Verification items for the finished model (mm, model axes). A direction names the side the tool comes from. Give positions to 0.01 mm unless a question says otherwise; leave off trailing zeros. Order: outer loops, then holes, each group sorted by start corner. A loop starts at its lowest first (then second) coordinate and runs counter-clockwise, first axis right, second up. Notation, with made-up numbers: (7, -2) - (51, -2) arc R32 cw to (51, 26) - close; hole circle Ø8 at (64.5, -3). An arc over 180 degrees is marked (long way). Answer as a JSON object with one key per item and string values. Group by question number.
(1) Thickness scan on line 1 (Z direction, x = 5.5, y = 39.3); line 2 (Z direction, x = 39, y = 3); line 3 (Y direction, x = 11, z = -11). Record the ranges inside material, lowest first.
(2) Access from +Z, -Z, +X, -X, +Y, -Y to the whole of each face (thin tool, end or side, straight path). Record for faces 1 (the face through (1.9, 36, 2)), 2 (the face through (21, 15, 2.4)), 3 (the face through (21, -2.4, -7)), 4 (the face through (21, 20, 0)), 5 (the face through (38.95, 40.28, 2.55)).
(3) Mould release check, pull along X, two halves, no side actions. Record for faces 6 (the face through (3.45, 40.28, 2.48)), 7 (the face through (40.5, 36, 2)), 8 (the face through (20.9, -1.8, 1.83)), 9 (the face through (10, 39, 2)): +X half, -X half, draft (parallel to the pull), parting line (faces both ways), or undercut.
(4) Section check B-B (x = 6). Record the boundary of the cut face in (y, z).
(5) Depth check by flat-ended pin: pin 1 Ø2 at (x, z) = (20, 2.5) entering from -Y; pin 2 Ø3.5 at (y, z) = (39, 3.5) entering from -X; pin 3 Ø10 at (x, z) = (23.5, -3.5) entering from +Y. Enter the tip coordinate at first touch or a pass-through.
(6) Section check A-A (z = 3.73). Record the boundary of the cut face in (x, y), then the cut area to 3 significant figures.
(7) Section check D-D (y = 5). Record the boundary of the cut face in (x, z), then the cut area to 3 significant figures.
(8) Section check C-C (x = 11). Record the boundary of the cut face in (y, z).
```python
from build123d import *

# Parameters (mm, degrees)
SKETCH1_W           = 42.4
SKETCH1_H           = 40.6
BOSS_EXTRUDE1_DEPTH = 2.4
SKETCH2_W           = 40
SKETCH2_H           = 2.4
BOSS_EXTRUDE2_DEPTH = 17.35
SKETCH3_W           = 22.4
SKETCH3_H           = 2.6
CUT_EXTRUDE1_DEPTH  = 2.4
BOSS_EXTRUDE3_DEPTH = 2.53
FILLET1_R           = 5.25
FILLET2_R           = 5.25
CUT_EXTRUDE2_DEPTH  = 16.4
FILLET3_R           = 2
CHAMFER1_SIZE       = 2
SKETCH9_W           = 1.9
SKETCH9_H           = 10
CUT_EXTRUDE4_DEPTH  = 61.577409156
FILLET5_R           = 2
BOSS_EXTRUDE4_DEPTH = 2.4
CUT_EXTRUDE5_START  = -8.1
SKETCH4_R           = 0.8255
CUT_EXTRUDE5_DEPTH  = 38.6


with BuildPart() as part:
    # Sketch1 → Boss-Extrude1 (new body)
    with BuildSketch(Plane.XY):
        with Locations((21.2, 20.3)):
            Rectangle(SKETCH1_W, SKETCH1_H)
    extrude(amount=BOSS_EXTRUDE1_DEPTH)

    # Sketch2 → Boss-Extrude2 (add)
    with BuildSketch(Plane.XY.offset(2.4)):
        with Locations((20, -1.2)):
            Rectangle(SKETCH2_W, SKETCH2_H)
    extrude(amount=-BOSS_EXTRUDE2_DEPTH)

    # Sketch3 → Cut-Extrude1 (cut)
    with BuildSketch(Plane.XY.offset(2.4)):
        with Locations((21.2, 39.3)):
            Rectangle(SKETCH3_W, SKETCH3_H)
    extrude(amount=-CUT_EXTRUDE1_DEPTH, mode=Mode.SUBTRACT)

    # Sketch5 → Boss-Extrude3 (add)
    with BuildSketch(Plane.XY.offset(2.4)):
        Polygon((0, 40.6), (0, 34.6), (42.4, 34.6), (42.4, 40.6), (32.4, 40.6), (32.4, 38), (10, 38), (10, 40.6), align=None)
    extrude(amount=BOSS_EXTRUDE3_DEPTH)

    # Fillet1
    fillet1_edges = [part.edges().sort_by_distance(p)[0] for p in [
        (0, 40.6, 2.465),
        (42.4, 40.6, 2.465),
    ]]
    fillet(fillet1_edges, radius=FILLET1_R)

    # Fillet2
    # the kernel refuses this fillet: 5.25 mm, written as the material it adds along each edge
    with BuildSketch(Plane(origin=(0, 34.6, 2.4), x_dir=(0, 0, 1), z_dir=(1, 0, 0))) as fillet2_piece_1:
        with BuildLine():
            CenterArc((5.25, 4.490445412), FILLET2_R, 180, 58.795429652)
            Line((0, 4.490445412), (-0.105, 4.490445412))
            Line((-0.105, 4.490445412), (-0.105, 0))
            Line((-0.105, 0), (0, -0.105))
            ThreePointArc((0, -0.105), (1.265, -0.105), (2.4756, -0.089808908))
            Line((2.4756, -0.089808908), (2.53, 0))
        make_face()
    extrude(amount=42.4)

    # Sketch6 → Cut-Extrude2 (cut)
    with BuildSketch(Plane.ZY.offset(-32.4)):
        Polygon((0, 40.6), (0, 38.6), (0.25, 40.6), align=None)
    cut_extrude2 = extrude(amount=-CUT_EXTRUDE2_DEPTH, mode=Mode.SUBTRACT)

    # Fillet3
    fillet3_edges = [part.edges().sort_by_distance(p)[0] for p in [
        (20, -2.4, 2.4),
    ]]
    fillet(fillet3_edges, radius=FILLET3_R)

    # Chamfer1
    chamfer1_edges = [part.edges().sort_by_distance(p)[0] for p in [
        (21.2, 38, 4.93),
    ]]
    chamfer(chamfer1_edges, length=CHAMFER1_SIZE)

    # Sketch9 → Cut-Extrude4 (cut, through all)
    with BuildSketch(Plane(origin=(0, 0, 0), x_dir=(-1, 0, 0), z_dir=(0, 0, -1))):
        with Locations((-41.45, 35.6)):
            Rectangle(SKETCH9_W, SKETCH9_H)
        with Locations((-0.95, 35.6)):
            Rectangle(SKETCH9_W, SKETCH9_H)
    extrude(amount=-CUT_EXTRUDE4_DEPTH, mode=Mode.SUBTRACT)

    # Fillet5
    # the kernel refuses this fillet: 2 mm, written as the material it adds along each edge
    with BuildSketch(Plane(origin=(1.9, 30.6, 0), x_dir=(0, 1, 0), z_dir=(0, 0, 1))) as fillet5_piece_1_section:
        with BuildLine():
            CenterArc((1.997498436, 2), FILLET5_R, 182.865983983, 87.134016017)
            Line((0, 1.9), (-0.039949969, 1.898))
            ThreePointArc((-0.039949969, 1.898), (-0.04, 0.95), (-0.04, 0))
            Line((-0.04, 0), (0, -0.04))
            Line((0, -0.04), (1.997498436, -0.04))
            Line((1.997498436, -0.04), (1.997498436, 0))
        make_face()
    fillet5_piece_1 = extrude(amount=7.416704545, mode=Mode.PRIVATE)
    fillet5_piece_1 = fillet5_piece_1 - Plane(origin=(1.464355644, 30.109554588, 7.65), x_dir=(0, 0, 1), z_dir=(-1, 0, 0)) * Cylinder(5.25, 23, mode=Mode.PRIVATE)
    add(fillet5_piece_1)
    with BuildSketch(Plane(origin=(40.5, 30.6, 0), x_dir=(0, 1, 0), z_dir=(0, 0, 1))) as fillet5_piece_2_section:
        with BuildLine():
            CenterArc((1.997498436, -2), FILLET5_R, 90, 87.134016017)
            Line((0, -1.9), (-0.039949969, -1.898))
            ThreePointArc((-0.039949969, -1.898), (-0.04, -0.95), (-0.04, 0))
            Line((-0.04, 0), (0, 0.04))
            Line((0, 0.04), (1.997498436, 0.04))
            Line((1.997498436, 0.04), (1.997498436, 0))
        make_face()
    fillet5_piece_2 = extrude(amount=7.416704545, mode=Mode.PRIVATE)
    fillet5_piece_2 = fillet5_piece_2 - Plane(origin=(40.935644356, 30.109554588, 7.65), x_dir=(0, 0, 1), z_dir=(-1, 0, 0)) * Cylinder(5.25, 23, mode=Mode.PRIVATE)
    add(fillet5_piece_2)

    # Sketch10 → Boss-Extrude4 (add)
    with BuildSketch(Plane(origin=(40, 0, 0), x_dir=(0, 0, -1), z_dir=(1, 0, 0))):
        with BuildLine():
            Line((-2.4, 0), (-2.4, -0.4))
            ThreePointArc((-2.4, -0.4), (-1.814213562, -1.814213562), (-0.4, -2.4))
            Line((-0.4, -2.4), (14.95, -2.4))
            Line((14.95, -2.4), (14.95, 0))
            Line((14.95, 0), (0, 0))
            Line((0, 0), (-2.4, 0))
        make_face()
    extrude(amount=BOSS_EXTRUDE4_DEPTH)

    # Mirror1: Cut-Extrude2 across plane
    add(cut_extrude2.mirror(Plane(origin=(21.2, 0, 0), x_dir=(0, 0, 1), z_dir=(1, 0, 0))), mode=Mode.SUBTRACT)

    # Sketch4 → Cut-Extrude5 (cut)
    with BuildSketch(Plane(origin=(10, 0, 0), x_dir=(0, 0, -1), z_dir=(1, 0, 0)).offset(CUT_EXTRUDE5_START)):
        with Locations(Location((-3.73, 39.3, 0), (0, 0, 173.581911643))):
            Circle(SKETCH4_R)
    extrude(amount=CUT_EXTRUDE5_DEPTH, mode=Mode.SUBTRACT)


solid = part.part
```
Solutions:
{
 "1": {"line 1": "z = 0.09 to 2.9, 4.56 to 4.93", "line 2": "z = 0 to 2.4", "line 3": "y = -2.4 to 0"},
 "2": {"face 1": "+Z, -Z, -X, +Y", "face 2": "+Z, +X, -X, -Y", "face 3": "+Z, -Z, +X, -X, -Y", "face 4": "-Z, +X, -X, +Y", "face 5": "+Z, -Z, +X, +Y"},
 "3": {"face 6": "-X half", "face 7": "+X half", "face 8": "draft", "face 9": "undercut"},
 "4": {"outline": "(-2.4, -14.95) - (0, -14.95) - (0, 0) - (38.6, 0) - (40.6, 0.25) - (40.6, 4.93) - (34.6, 4.93) arc R5.25 cw to (30.11, 2.4) - (-0.4, 2.4) arc R2 ccw to (-2.4, 0.4) - close; hole circle Ø1.65 at (39.3, 3.73)"},
 "5": {"pin 1": "stops at y = -2.07", "pin 2": "stops at x = 1.9", "pin 3": "stops at y = 38"},
 "6": {"outline": "(1.9, 33.6) - (40.5, 33.6) - (40.5, 38.47) - (32.4, 38.47) - (32.4, 37.2) - (10, 37.2) - (10, 38.47) - (1.9, 38.47) - close; (3.07, 40.13) - (10, 40.13) - (10, 40.6) - (5.25, 40.6) arc R5.25 ccw to start; (32.4, 40.13) - (39.33, 40.13) arc R5.25 ccw to (37.15, 40.6) - (32.4, 40.6) - close", "area": "165 mm2"},
 "7": {"outline": "(0, 0) - (42.4, 0) - (42.4, 2.4) - (0, 2.4) - close", "area": "102 mm2"},
 "8": {"outline": "(-2.4, -14.95) - (0, -14.95) - (0, 0) - (38, 0) - (38, 2.93) - (36, 4.93) - (34.6, 4.93) arc R5.25 cw to (30.11, 2.4) - (-0.4, 2.4) arc R2 ccw to (-2.4, 0.4) - close"}
}
